For this review, take the finished solid that the model builds, in its own axes (mm). A direction names the side the tool comes from. Coordinates: 2 decimals unless noted, no trailing zeros. Write each loop counter-clockwise with the first axis right and the second up, starting at its lowest first coordinate (ties: lowest second). Pieces come first, ordered by that corner, then holes.
```python
from build123d import *

# Parameters (mm, degrees)
SKETCH_1_W          = 169
SKETCH_1_H          = 41
EXTRUDE_2_DEPTH     = 5
SKETCH_3_R          = 1.5
CUT_EXTRUDE_1_DEPTH = 5
SKETCH_4_W          = 169
SKETCH_4_H          = 26
EXTRUDE_3_DEPTH     = 20
SKETCH_5_W          = 20
SKETCH_5_H          = 21
CUT_EXTRUDE_2_DEPTH = 55
SKETCH_6_W          = 20
SKETCH_6_H          = 21
CUT_EXTRUDE_3_DEPTH = 55
CUT_EXTRUDE_6_DEPTH = 59
SKETCH_10_W         = 7.7
SKETCH_10_H         = 21
CUT_EXTRUDE_7_DEPTH = 59
SKETCH_11_W         = 4
SKETCH_11_H         = 15
CUT_EXTRUDE_8_DEPTH = 59


with BuildPart() as part:
    # Эскиз1 → Бобышка-Вытянуть2 (new body)
    with BuildSketch(Plane.XY):
        Rectangle(SKETCH_1_W, SKETCH_1_H)
    extrude(amount=EXTRUDE_2_DEPTH)

    # Эскиз3 → Вырез-Вытянуть1 (cut)
    with BuildSketch(Plane.XY.offset(5)):
        with Locations((79.5, 16.5)):
            Circle(SKETCH_3_R)
        with Locations((34.5, 16.5)):
            Circle(SKETCH_3_R)
        with Locations((-34.5, 16.5)):
            Circle(SKETCH_3_R)
        with Locations((-79.5, 16.5)):
            Circle(SKETCH_3_R)
    extrude(amount=-CUT_EXTRUDE_1_DEPTH, mode=Mode.SUBTRACT)

    # Эскиз4 → Бобышка-Вытянуть3 (add)
    with BuildSketch(Plane.XY.offset(5)):
        with Locations((0, -7.5)):
            Rectangle(SKETCH_4_W, SKETCH_4_H)
    extrude(amount=EXTRUDE_3_DEPTH)

    # Эскиз5 → Вырез-Вытянуть2 (cut)
    with BuildSketch(Plane.ZY.offset(84.5)):
        with Locations((15, -7.5)):
            Rectangle(SKETCH_5_W, SKETCH_5_H)
    extrude(amount=-CUT_EXTRUDE_2_DEPTH, mode=Mode.SUBTRACT)

    # Эскиз6 → Вырез-Вытянуть3 (cut)
    with BuildSketch(Plane(origin=(84.5, 0, 0), x_dir=(0, 0, -1), z_dir=(1, 0, 0))):
        with Locations((-15, -7.5)):
            Rectangle(SKETCH_6_W, SKETCH_6_H)
    extrude(amount=-CUT_EXTRUDE_3_DEPTH, mode=Mode.SUBTRACT)

    # Эскиз7 → Вырез-Вытянуть6 (cut)
    with BuildSketch(Plane(origin=(29.5, 0, 0), x_dir=(0, 0, -1), z_dir=(1, 0, 0))):
        with BuildLine():
            Line((-5, 3), (-10.3, 3))
            ThreePointArc((-10.3, 3), (-12.421320344, 2.121320344), (-13.3, 0))
            Line((-13.3, 0), (-13.3, -15))
            ThreePointArc((-13.3, -15), (-12.421320344, -17.121320344), (-10.3, -18))
            Line((-10.3, -18), (-5, -18))
            Line((-5, -18), (-5, 3))
        make_face()
    extrude(amount=-CUT_EXTRUDE_6_DEPTH, mode=Mode.SUBTRACT)

    # Эскиз10 → Вырез-Вытянуть7 (cut)
    with BuildSketch(Plane(origin=(29.5, 0, 0), x_dir=(0, 0, -1), z_dir=(1, 0, 0))):
        with Locations((-21.15, -7.5)):
            Rectangle(SKETCH_10_W, SKETCH_10_H)
    extrude(amount=-CUT_EXTRUDE_7_DEPTH, mode=Mode.SUBTRACT)

    # Эскиз11 → Вырез-Вытянуть8 (cut)
    with BuildSketch(Plane(origin=(29.5, 0, 0), x_dir=(0, 0, -1), z_dir=(1, 0, 0))):
        with Locations((-15.3, -7.5)):
            Rectangle(SKETCH_11_W, SKETCH_11_H)
    extrude(amount=-CUT_EXTRUDE_8_DEPTH, mode=Mode.SUBTRACT)


solid = part.part
```
Q1. Add section A-A (x = -79.5). State the section outline as (y, z) points.
Ans:
outline: (-20.5, 0) - (15, 0) - (15, 5) - (5.5, 5) - (5.5, 25) - (3, 25) - (3, 5) - (-18, 5) - (-18, 25) - (-20.5, 25) - close; (18, 0) - (20.5, 0) - (20.5, 5) - (18, 5) - close
Q2. Draft analysis for pull direction Y (two halves, no side actions). For faces 1 (the flat face through (-1, 5.5, 15)), 2 (the flat face through (-1, -20.5, 12)), 3 (the cylindrical face through (-35.61, 17.51, 2.54)), 4 (the flat face through (-1, 13, 5)), state which applies: +Y half, -Y half, draft (parallel to the pull), parting line (faces both ways), or undercut.
Ans:
face 1: +Y half
face 2: -Y half
face 3: undercut
face 4: draft
Q3. Add section B-B (y = 16.5). State the section outline as (x, z) points, then the cut area to 3 significant figures.
Ans:
outline: (-84.5, 0) - (-81, 0) - (-81, 5) - (-84.5, 5) - close; (-78, 0) - (-36, 0) - (-36, 5) - (-78, 5) - close; (-33, 0) - (33, 0) - (33, 5) - (-33, 5) - close; (36, 0) - (78, 0) - (78, 5) - (36, 5) - close; (81, 0) - (84.5, 0) - (84.5, 5) - (81, 5) - close
area: 785 mm2
Q4. For probe 1 along Y at (x, z) = (-47, 6.5); probe 2 along Y at (x, z) = (79.5, 3.1); probe 3 along Z at (x, y) = (0.5, 1), list the stretches that pass through material, from the lowest coordinate up.
Ans:
probe 1: y = -20.5 to -18, 3 to 5.5
probe 2: y = -20.5 to 15, 18 to 20.5
probe 3: z = 0 to 5, 13.13 to 17.3
Q5. Add section D-D (x = -46). State the section outline as (y, z) points.
Ans:
outline: (-20.5, 0) - (20.5, 0) - (20.5, 5) - (5.5, 5) - (5.5, 25) - (3, 25) - (3, 5) - (-18, 5) - (-18, 25) - (-20.5, 25) - close
Q6. Tool access review of faces 5 (the flat face through (-29.5, -16, 15)), 6 (the flat face through (0, 0, 15)), 7 (the cylindrical face through (0.41, -17.1, 12.44)), 8 (the flat face through (29.5, 2, 15)): name each direction out of +Z, -Z, +X, -X, +Y, -Y from which nothing blocks a thin tool from reaching the whole face with its end or side.
Ans:
face 5: +Z, -X
face 6: +Z, +X, -X
face 7: +X, -X
face 8: +Z, +X
Q7. Add section C-C (z = 14.75). State the section outline as (x, y) points, then the cut area to 3 significant figures.
Ans:
outline: (-84.5, -20.5) - (84.5, -20.5) - (84.5, -18) - (29.5, -18) - (29.5, -15) - (-29.5, -15) - (-29.5, -18) - (-84.5, -18) - close; (-84.5, 3) - (-29.5, 3) - (-29.5, 0) - (29.5, 0) - (29.5, 3) - (84.5, 3) - (84.5, 5.5) - (-84.5, 5.5) - close
area: 1,200 mm2
Q8. Clearance check with flat-ended pins moving along their axes: pin 1 Ø12 at (x, y) = (24, 12) entering from +Z; pin 2 Ø1.5 at (y, z) = (-16, 13) entering from +X; pin 3 Ø2 at (x, z) = (-5.5, 15) entering from +Y. State where each tip first meets the part, or that it passes through.
Ans:
pin 1: stops at z = 5
pin 2: stops at x = 29.5
pin 3: stops at y = 5.5
